Check sheet for the modelled part. Datum: model origin and axes. Units: mm. A direction names the side the tool comes from. Coordinates: 2 decimals unless noted, no trailing zeros. Loops run counter-clockwise (first coordinate to the right, second up) from the corner with the lowest first, then second, coordinate; pieces in that order, holes last. Notation, with made-up numbers: (-8, -27.5) -> (29, -27.5) arc R19 ccw to (29, -1.5) -> close; hole circle Ø3 at (32.5, 25). An arc over 180 degrees is marked (long way). Use one line per item in the form item = value.
from build123d import *

# Parameters (mm, degrees)
F0_W      = 272
F0_H      = 19.490359351
F0_H_2    = 30.509640649
F1_DEPTH  = 6
F2_D      = 11
F3_D      = 11
F4_D      = 9.2
F5_D      = 8
F6_D      = 7
F7_D      = 6
F8_D      = 6
F9_D      = 6
F10_DEPTH = 50
F11_W     = 272
F11_H     = 5
F12_DEPTH = 50


with BuildPart() as f1:
    # F0 (on Top) → F1 (new body)
    with BuildSketch(Plane.XY):
        with Locations((-83.9492530227, -9.7451796755)):
            Rectangle(F0_W, F0_H)
        with Locations((-83.9492530227, 15.2548203245)):
            Rectangle(F0_W, F0_H_2)
    extrude(amount=-F1_DEPTH)

    # F2 (through all)
    with Locations(Plane.XY):
        with Locations((-193.9492530227, 0)):
            Hole(F2_D / 2)

    # F3 (through all)
    with Locations(Plane.XY):
        with Locations((-158.9492530227, 0)):
            Hole(F3_D / 2)

    # F4 (through all)
    with Locations(Plane.XY):
        with Locations((-126.4492530227, 0)):
            Hole(F4_D / 2)

    # F5 (through all)
    with Locations(Plane.XY):
        with Locations((-93.9492530227, 0)):
            Hole(F5_D / 2)

    # F6 (through all)
    with Locations(Plane.XY):
        with Locations((-61.5492530227, 0)):
            Hole(F6_D / 2)

    # F7 (through all)
    with Locations(Plane.XY):
        with Locations((-30.4492530227, 0)):
            Hole(F7_D / 2)

    # F8 (through all)
    with Locations(Plane.XY):
        with Locations((29.0007469773, 0)):
            Hole(F8_D / 2)

    # F9 (through all)
    with Locations(Plane.XY):
        with Locations((-0.6492530227, 0)):
            Hole(F9_D / 2)

    # F10 (add): a face of the model
    f10_faces = [f1.faces().sort_by_distance(p)[0] for p in [
        (-83.9492530227, 30.509640649, -3),
    ]]
    extrude(f10_faces, amount=F10_DEPTH)

    # F11 (on face) → F12 (join)
    with BuildSketch(Plane.XY):
        with Locations((-83.9492530227, 78.009640649)):
            Rectangle(F11_W, F11_H)
    extrude(amount=F12_DEPTH)


solid = f1.part
(1) Section check A-A, the plane x = -103. Record the boundary of the cut face in (y, z), plus the area to 3 significant figures.
Established:
outline = (-19.49, -6) -> (80.51, -6) -> (80.51, 50) -> (75.51, 50) -> (75.51, 0) -> (-19.49, 0) -> close
area = 850 mm²
(2) Go/stop test with flat-tipped pins: P1, Ø8, axis at x = -0.65, y = 0, coming from the +Z side; P2, Ø12, axis at x = -84.5, z = 44, coming from the -Y side. Record where each tip stops, or that it passes through.
Established:
P1 = 0
P2 = 75.51
(3) Mould release check, pull along X, two halves, no side actions. Record for faces 1 (the flat face through (52.051, 38, -1)), 2 (the cylindrical face through (-64.8, -1.3, -3)), 3 (the cylindrical face through (-89.953, 0.176, -3.042)), 4 (the flat face through (-86, 80.51, 22)): +X half, -X half, draft (parallel to the pull), parting line (faces both ways), or undercut.
Established:
face_1 = +X half
face_2 = undercut
face_3 = undercut
face_4 = draft
(4) Tool access check on faces 5 (the cylindrical face through (2.348, 0.132, -3.042)), 6 (the flat face through (-86, 75.51, 25)). Record the directions out of +Z, -Z, +X, -X, +Y, -Y that give a thin tool (end or side, any length) a straight path to the whole face; none if there is none.
Established:
face_5 = +Z, -Z
face_6 = +Z, +X, -X, -Y
(5) Scan lines: line 1 along Y through (x, z) = (-0.5, -3); line 2 along Y through (x, z) = (24.5, 45); line 3 along Z through (x, y) = (-92.5, 30.5). Record each from-to range of solid material in increasing order.
Established:
line_1 = -19.49 to -3, 3 to 80.51
line_2 = 75.51 to 80.51
line_3 = -6 to 0
(6) Section check D-D, the plane y = 59.5. Record the boundary of the cut face in (x, z), plus the area to 3 significant figures.
Established:
outline = (-219.95, -6) -> (52.05, -6) -> (52.05, 0) -> (-219.95, 0) -> close
area = 1,630 mm²
(7) Section check B-B, the plane y = 0. Give the number of separate pieces and of enclosed holes in the cut face, plus the area to 3 significant figures.
Established:
separate_pieces = 9
enclosed_holes = 0
area = 1,250 mm²
(8) Section check C-C, the plane z = 35. Record the boundary of the cut face in (x, y).
Established:
outline = (-219.95, 75.51) -> (52.05, 75.51) -> (52.05, 80.51) -> (-219.95, 80.51) -> close
